Could you check a few things on this model? Use its own coordinates, in mm. Face numbers are marked on the shaded views. Give positions to 0.01 mm unless a question says otherwise; leave off trailing zeros. Order: outer loops, then holes, each group sorted by start corner. A loop starts at its lowest first (then second) coordinate and runs counter-clockwise, first axis right, second up. Notation, with made-up numbers: (44.25, 66.5) - (88.25, 66.5) arc R20 cw to (88.25, 74.5) - close; hole circle Ø11 at (43, 76). An arc over 180 degrees is marked (long way). Put each result on its own line as item: value.
from build123d import *

# Parameters (mm, degrees)
F0_R     = 6.35
F5_DEPTH = 19.05
F1_R     = 5.08
F4_R     = 2.8448
F7_R     = 6.35
F7_R_2   = 4.445
F8_DEPTH = 12.7


with BuildPart() as f5:
    # F0 (on Front) → F5 (new body)
    with BuildSketch(Plane.XZ):
        Circle(F0_R)
    extrude(amount=-F5_DEPTH)

    # F1 (on face) → F6 section 0
    with BuildSketch(Plane.XZ):
        Circle(F1_R)
    # F4 (on line) → F6 section 1
    with BuildSketch(Plane(origin=(0, 19.05, 0), x_dir=(-1, 0, 0), z_dir=(0, 1, 0))):
        Circle(F4_R)
    loft(mode=Mode.SUBTRACT)

    # F7 (on face) → F8 (join)
    with BuildSketch(Plane(origin=(0, 19.05, 0), x_dir=(-1, 0, 0), z_dir=(0, 1, 0))):
        Circle(F7_R)
        Circle(F7_R_2, mode=Mode.SUBTRACT)
    extrude(amount=F8_DEPTH)


solid = f5.part
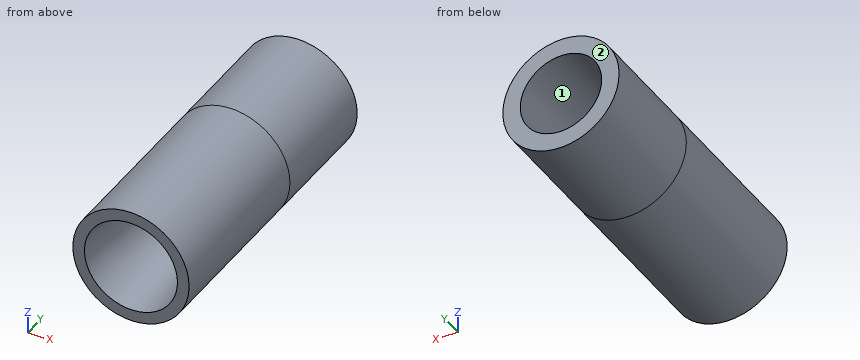
1) If I drill on line 1 (Z direction, x = 0, y = 22) (3 decimals); line 2 (Z direction, x = 0, y = 17); line 3 (X direction, y = 20, z = -3), over which ranges is the centre line in solid material (lowest first)? Write a range as [from, to].
Filled in:
line 1: z = [-6.35, -4.445], [4.445, 6.35]
line 2: z = [-6.35, -3.09], [3.09, 6.35]
line 3: x = [-5.6, -3.28], [3.28, 5.6]
2) We'd pull the mould along Z, two halves only. Please class the marked faces 1 and 2: pulls with the +Z half, pulls with the -Z half, needs draft (parallel to the pull), parting line crosses it, or undercut.
Filled in:
face 1: undercut
face 2: needs draft
3) I'm going to push flat-ended pins straight in: pin 1 (5 mm diameter, centred on x = 1, y = 21, fed in from +Z); pin 2 (5.5 mm diameter, centred on x = 0, z = 0, fed in from +Y); pin 3 (4 mm diameter, centred on x = 3.5, y = 15.5, fed in from +Z); pin 4 (2.5 mm diameter, centred on x = 1, z = 2, fed in from +Y). Where does each tip first touch, or does it pass through?
Filled in:
pin 1: stops at z = 6.35
pin 2: passes through
pin 3: stops at z = 6.17
pin 4: stops at y = 19.05
4) Suppose I cut it at A-A, the plane x = 0. List the corners of the cut face in (y, z) for me (3 decimals).
Filled in:
outline: (0, -6.35) - (31.75, -6.35) - (31.75, -4.445) - (19.05, -4.445) - (19.05, -2.845) - (0, -5.08) - close; (0, 5.08) - (19.05, 2.845) - (19.05, 4.445) - (31.75, 4.445) - (31.75, 6.35) - (0, 6.35) - close
5) Suppose I cut it at C-C, the plane y = 18. List the corners of the cut face in (x, z) for me.
Filled in:
outline: circle Ø12.7 at (0, 0); hole circle Ø5.94 at (0, 0)
6) Suppose I cut it at B-B, the plane y = 23. List the corners of the cut face in (x, z) for me (3 decimals).
Filled in:
outline: circle Ø12.7 at (0, 0); hole circle Ø8.89 at (0, 0)
